```python
from build123d import *

# Parameters (mm, degrees)
SKETCH1_R               = 27.5
SKETCH1_R_2             = 22.5
BOSS_EXTRUDE1_DEPTH     = 5
CUT_EXTRUDE3_DEPTH      = 28.5
CUT_EXTRUDE3_DEPTH_BACK = 28.5


with BuildPart() as part:
    # Sketch1 → Boss-Extrude1 (new body, symmetric)
    with BuildSketch(Plane(origin=(0, 0, 0), x_dir=(1, 0, 0), z_dir=(0, 1, 0))):
        Circle(SKETCH1_R)
        Circle(SKETCH1_R_2, mode=Mode.SUBTRACT)
    extrude(amount=BOSS_EXTRUDE1_DEPTH, both=True)

    # Sketch3 → Cut-Extrude3 (cut, two sides)
    with BuildSketch(Plane.XY) as cut_extrude3_sk:
        with BuildLine():
            ThreePointArc((-4.74745791, 0.318346798), (-3.065358978, -2.467655845), (0, -3.56074408))
            Line((0, -3.56074408), (0, 5))
            Line((0, 5), (-20.700497525, 5))
            Line((-20.700497525, 5), (-20.700497525, 2.615010963))
            ThreePointArc((-20.700497525, 2.615010963), (-18.866910307, 1.311744504), (-16.85614269, 2.320386731))
            ThreePointArc((-16.85614269, 2.320386731), (-14.987432042, 3.204610911), (-13.38889815, 1.893648941))
            ThreePointArc((-13.38889815, 1.893648941), (-11.548514755, 0.343661099), (-9.334889148, 1.286706711))
            ThreePointArc((-9.334889148, 1.286706711), (-6.723222767, 2.308761406), (-4.74745791, 0.318346798))
        make_face()
        with BuildLine():
            Line((0, 5), (0, -3.56074408))
            ThreePointArc((0, -3.56074408), (3.065358978, -2.467655845), (4.74745791, 0.318346798))
            ThreePointArc((4.74745791, 0.318346798), (6.723222767, 2.308761406), (9.334889148, 1.286706711))
            ThreePointArc((9.334889148, 1.286706711), (11.548514755, 0.343661099), (13.38889815, 1.893648941))
            ThreePointArc((13.38889815, 1.893648941), (14.987432042, 3.204610911), (16.85614269, 2.320386731))
            ThreePointArc((16.85614269, 2.320386731), (18.866910307, 1.311744504), (20.700497525, 2.615010963))
            Line((20.700497525, 2.615010963), (20.700497525, 5))
            Line((20.700497525, 5), (0, 5))
        make_face()
    extrude(amount=CUT_EXTRUDE3_DEPTH, mode=Mode.SUBTRACT)
    extrude(cut_extrude3_sk.sketch, amount=-CUT_EXTRUDE3_DEPTH_BACK, mode=Mode.SUBTRACT)


solid = part.part
```
The listing builds one solid part. Answer for the finished solid, in the listing's coordinates (mm). A direction names the side the tool comes from. Coordinates: 2 decimals unless noted, no trailing zeros. Write each loop counter-clockwise with the first axis right and the second up, starting at its lowest first coordinate (ties: lowest second). Pieces come first, ordered by that corner, then holes.
Q1. Section D-D, the plane z = -9.5 is taken. Write down the section's boundary in (x, y) (1 decimal), then the cut area to 3 significant figures.
Returned:
outline: (-25.8, -5) - (-20.4, -5) - (-20.4, 2.1) arc R2.2 cw to (-20.7, 2.6) - (-20.7, 5) - (-25.8, 5) - close; (20.4, -5) - (25.8, -5) - (25.8, 5) - (20.7, 5) - (20.7, 2.6) arc R2.2 cw to (20.4, 2.1) - close
area: 107 mm2
Q2. Section B-B, the plane z = 2 is taken. Write down the section's boundary in (x, y).
Returned:
outline: (-27.43, -5) - (-22.41, -5) - (-22.41, 5) - (-27.43, 5) - close; (22.41, -5) - (27.43, -5) - (27.43, 5) - (22.41, 5) - close
Q3. The mould has two halves that part along X. Classify faces 3 (the cylindrical face through (-11.58, 0.35, 21.92)), 4 (the cylindrical face through (12.69, -1.041, 24.397)), 5 (the flat face through (-23, -5, 0)): released by +X, released by -X, zero draft, split by the parting line, or undercut.
Returned:
face 3: undercut
face 4: split by the parting line
face 5: zero draft
Q4. Section A-A, the plane y = 4 is taken. Write down the section's boundary in (x, z), then the cut area to 3 significant figures.
Returned:
outline: (-20.7, -18.1) - (-20.7, -8.82) arc R22.5 cw to (-20.7, 8.82) - (-20.7, 18.1) arc R27.5 ccw to start; (20.7, -18.1) arc R27.5 ccw to (20.7, 18.1) - (20.7, 8.82) arc R22.5 cw to (20.7, -8.82) - close
area: 295 mm2
Q5. Find the intervals of material crossed by line 1 along X through (y, z) = (-2.25, 0); line 2 along X through (y, z) = (0.5, 24); line 3 along X through (y, z) = (-2, 11.5), in increasing order.
Returned:
line 1: x = -27.5 to -22.5, 22.5 to 27.5
line 2: x = -13.43 to -12.1, -10.31 to -4.79, 4.79 to 10.31, 12.1 to 13.43
line 3: x = -24.98 to -19.34, 19.34 to 24.98
Q6. Given P1, Ø2.5, axis at y = 4, z = 12.5, coming from the -X side; P2, Ø1, axis at x = 9.5, y = 0.5, coming from the -Z side; P3, Ø1.2, axis at y = 4, z = 14.5, coming from the +X side; P4, Ø10, axis at x = -6.5, z = -14.5, coming from the +Y side, each flat-ended and moving along its own axis, determine where each tip first touches the part or whether it passes through.
Returned:
P1: stops at x = -25.09
P2: stops at z = -25.99
P3: stops at x = 23.73
P4: passes through
Q7. Section C-C, the plane z = 14 is taken. Write down the section's boundary in (x, y) (1 decimal), then the cut area to 4 significant figures.
Returned:
outline: (-23.7, -5) - (-17.6, -5) - (-17.6, 1.6) arc R2.2 cw to (-20.7, 2.6) - (-20.7, 5) - (-23.7, 5) - close; (17.6, -5) - (23.7, -5) - (23.7, 5) - (20.7, 5) - (20.7, 2.6) arc R2.2 cw to (17.6, 1.6) - close
area: 100.0 mm2
Q8. Which of the six approach directions +Z, -Z, +X, -X, +Y, -Y give full straight-line access (tool end or side, diameter ignored) to faces 1 (the flat face through (-20.7, 4, 13)), 2 (the flat face through (-23, 5, 0))?
Returned:
face 1: +Z, -Z, +Y
face 2: +Z, -Z, +X, -X, +Y
